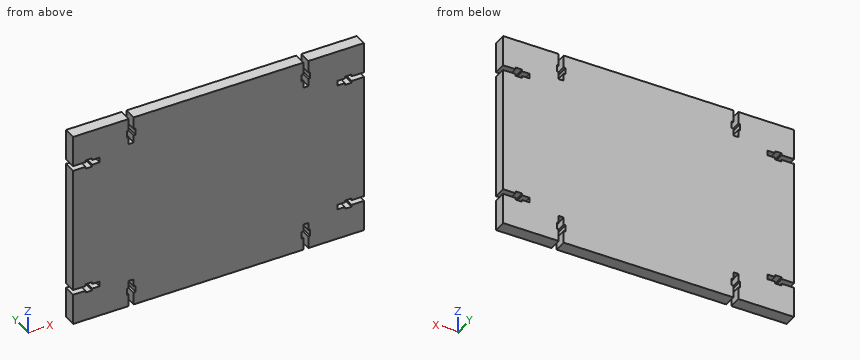
from build123d import *

# Parameters (mm, degrees)
SKETCH1_W               = 235
SKETCH1_H               = 10
BOSS_EXTRUDE1_DEPTH     = 160
ENL_V_MAT_EXTRU_2_DEPTH = 10
ENL_V_MAT_EXTRU_3_DEPTH = 10


with BuildPart() as part:
    # Sketch1 → Boss-Extrude1 (new body)
    with BuildSketch(Plane.XY):
        with Locations((117.5, 5)):
            Rectangle(SKETCH1_W, SKETCH1_H)
    extrude(amount=BOSS_EXTRUDE1_DEPTH)

    # Esquisse2 → Enlèv. mat.-Extru.2 (cut)
    with BuildSketch(Plane.XZ):
        Polygon((0, 135), (10, 135), (10, 136.55), (15.5, 136.55), (15.5, 135), (21.5, 135), (21.5, 131), (15.5, 131), (15.5, 129.45), (10, 129.45), (10, 131), (0, 131), align=None)
        Polygon((0, 29), (10, 29), (10, 30.55), (15.5, 30.55), (15.5, 29), (21.5, 29), (21.5, 25), (15.5, 25), (15.5, 23.45), (10, 23.45), (10, 25), (0, 25), align=None)
        Polygon((235, 25), (225, 25), (225, 23.45), (219.5, 23.45), (219.5, 25), (213.5, 25), (213.5, 29), (219.5, 29), (219.5, 30.55), (225, 30.55), (225, 29), (235, 29), align=None)
        Polygon((235, 131), (225, 131), (225, 129.45), (219.5, 129.45), (219.5, 131), (213.5, 131), (213.5, 135), (219.5, 135), (219.5, 136.55), (225, 136.55), (225, 135), (235, 135), align=None)
    extrude(amount=-ENL_V_MAT_EXTRU_2_DEPTH, mode=Mode.SUBTRACT)

    # Esquisse3 → Enlèv. mat.-Extru.3 (cut)
    with BuildSketch(Plane.XZ):
        Polygon((45, 160), (45, 150), (43.45, 150), (43.45, 144.5), (45, 144.5), (45, 138.5), (49, 138.5), (49, 144.5), (50.55, 144.5), (50.55, 150), (49, 150), (49, 160), align=None)
        Polygon((186, 160), (186, 150), (184.45, 150), (184.45, 144.5), (186, 144.5), (186, 138.5), (190, 138.5), (190, 144.5), (191.55, 144.5), (191.55, 150), (190, 150), (190, 160), align=None)
        Polygon((190, 0), (190, 10), (191.55, 10), (191.55, 15.5), (190, 15.5), (190, 21.5), (186, 21.5), (186, 15.5), (184.45, 15.5), (184.45, 10), (186, 10), (186, 0), align=None)
        Polygon((49, 0), (49, 10), (50.55, 10), (50.55, 15.5), (49, 15.5), (49, 21.5), (45, 21.5), (45, 15.5), (43.45, 15.5), (43.45, 10), (45, 10), (45, 0), align=None)
    extrude(amount=-ENL_V_MAT_EXTRU_3_DEPTH, mode=Mode.SUBTRACT)


solid = part.part
Part model, mm, in its own coordinate system. Round coordinates to 2 decimals unless told otherwise and drop trailing zeros. Loops run counter-clockwise (first coordinate to the right, second up) from the corner with the lowest first, then second, coordinate; pieces in that order, holes last. Notation, with made-up numbers: (-10.5, -27.75) - (11.5, -27.75) arc R18 ccw to (11.5, -12.75) - close; hole circle Ø5 at (22, 5.25). An arc over 180 degrees is marked (long way). Answer as a JSON object with one key per item and string values.
Item 1: Wall check: L1, parallel to Z at x = 10.5, y = 5; L2, parallel to X at y = 4.5, z = 143.5; L3, parallel to X at y = 8.25, z = 136.5. Give the ranges that are in metal, low to high.
Output:
{"L1": "0 to 23.45, 30.55 to 129.45, 136.55 to 160", "L2": "0 to 45, 49 to 186, 190 to 235", "L3": "0 to 10, 15.5 to 219.5, 225 to 235"}
Item 2: Band-saw the part on A-A on z = 18.5. List the corners of the cut face in (x, y), plus the area to 3 significant figures.
Output:
{"outline": "(0, 0) - (45, 0) - (45, 10) - (0, 10) - close; (49, 0) - (186, 0) - (186, 10) - (49, 10) - close; (190, 0) - (235, 0) - (235, 10) - (190, 10) - close", "area": "2,270 mm2"}
Item 3: Pin check, flat tips, straight feed: pin 1 (1 mm diameter, centred on x = 109, z = 121, fed in from -Y); pin 2 (2 mm diameter, centred on x = 188.5, y = 6.5, fed in from -Z); pin 3 (1.2 mm diameter, centred on y = 4, z = 132, fed in from +X). Stop position of each tip, or through.
Output:
{"pin 1": "y = 0", "pin 2": "z = 21.5", "pin 3": "x = 213.5"}
